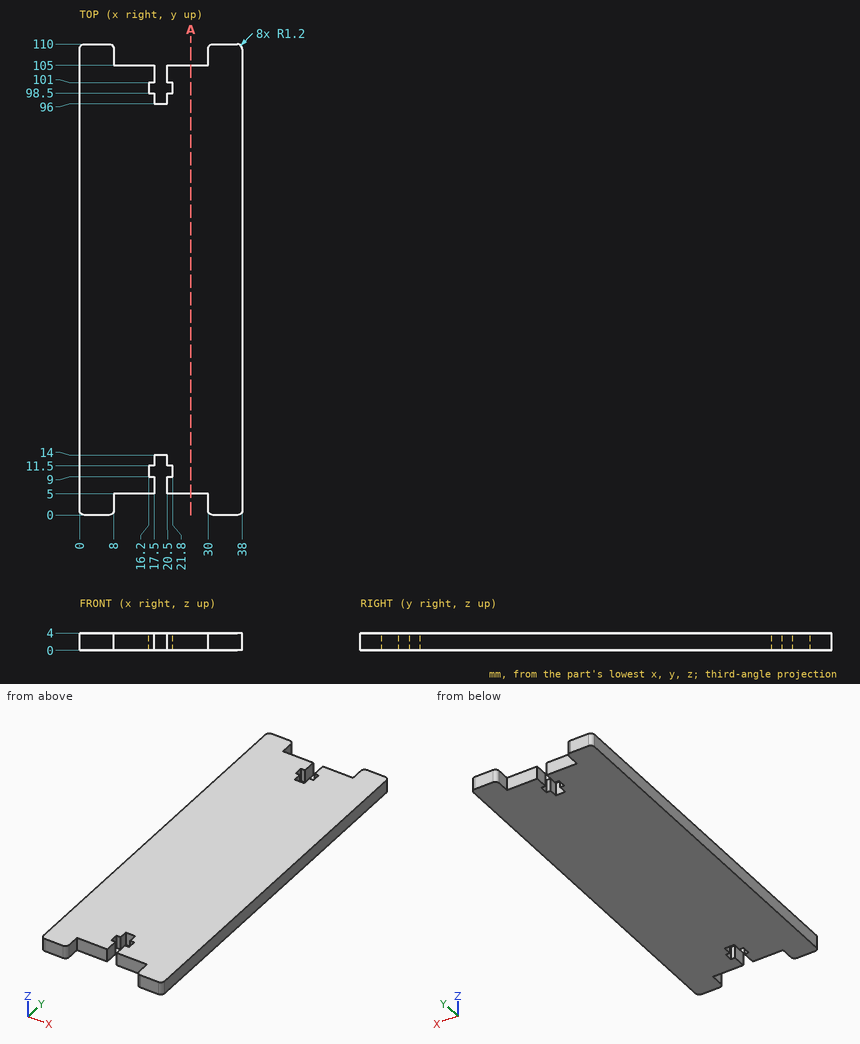
Check sheet for the drawn part. Datum: minimum x, y, z corner. Units: mm. Give positions to 0.01 mm unless a question says otherwise; leave off trailing zeros. Order: outer loops, then holes, each group sorted by start corner. A loop starts at its lowest first (then second) coordinate and runs counter-clockwise, first axis right, second up.
1. Sectioned sample at A-A (x = 26). Record the boundary of the cut face in (y, z).
Completed:
outline: (5, 0) - (105, 0) - (105, 4) - (5, 4) - close
2. Depth check by flat-ended pin: pin 1 (1.2 mm diameter, centred on x = 25, z = 2.5, fed in from -Y); pin 2 (0.7 mm diameter, centred on x = 17, z = 1.5, fed in from +Y); pin 3 (1.5 mm diameter, centred on x = 19.5, z = 1, fed in from +Y). Enter the tip coordinate at first touch or a pass-through.
Completed:
pin 1: stops at y = 5
pin 2: stops at y = 105
pin 3: stops at y = 96
3. Scan lines: line 1 (X direction, y = 10, z = 0.55); line 2 (X direction, y = 12, z = 2.6); line 3 (Y direction, x = 27.5, z = 0.85). Record each from-to range of solid material in increasing order.
Completed:
line 1: x = 0 to 16.2, 21.8 to 38
line 2: x = 0 to 17.5, 20.5 to 38
line 3: y = 5 to 105
